```python
from build123d import *

# Parameters (mm, degrees)
BOSS_EXTRUDE1_DEPTH = 1.524


with BuildPart() as part:
    # Sketch1 → Boss-Extrude1 (new body)
    with BuildSketch(Plane.XY):
        with BuildLine():
            ThreePointArc((12.566304874, -9.8933052), (12.77131161, -10.004957793), (12.965201909, -10.13496016))
            ThreePointArc((12.965201909, -10.13496016), (18.14143902, -15.472865183), (21.320013307, -22.194719552))
            ThreePointArc((21.320013307, -22.194719552), (20.806583347, -23.173609324), (19.854339012, -22.612301713))
            ThreePointArc((19.854339012, -22.612301713), (16.93227249, -16.403886417), (12.182265789, -11.452085777))
            ThreePointArc((12.182265789, -11.452085777), (11.989118214, -11.3205608), (11.784700698, -11.207342939))
            ThreePointArc((11.784700698, -11.207342939), (5.914450191, -6.588756496), (2.396003148, 0))
            Line((2.396003148, 0), (3.20554689, 0))
            Line((3.20554689, 0), (3.20554689, 1.524))
            Line((3.20554689, 1.524), (4.72954689, 1.524))
            Line((4.72954689, 1.524), (4.72954689, 0))
            Line((4.72954689, 0), (5.480406076, 0))
            ThreePointArc((5.480406076, 0), (5.996385034, -3.275905029), (7.587657532, -6.185482298))
            ThreePointArc((7.587657532, -6.185482298), (9.902770623, -8.273313508), (12.566304874, -9.8933052))
        make_face()
    extrude(amount=BOSS_EXTRUDE1_DEPTH)


solid = part.part
```
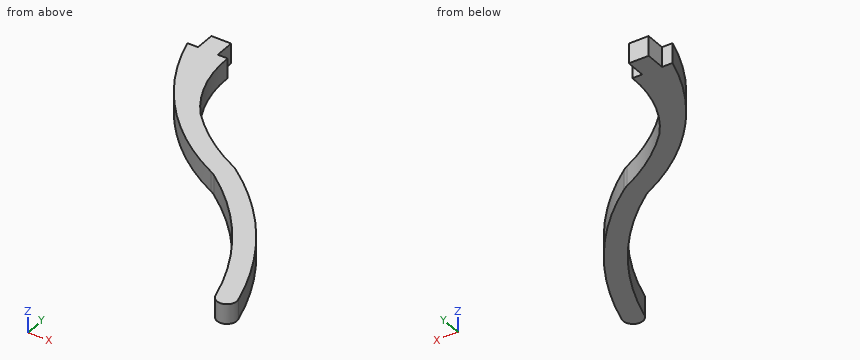
CAD build for the part. Positions are in the model's coordinates, mm. Coordinates: 2 decimals unless noted, no trailing zeros. Order: outer loops, then holes, each group sorted by start corner. A loop starts at its lowest first (then second) coordinate and runs counter-clockwise, first axis right, second up.
(1) Saw through at C-C, the plane y = -18.5. Write the cut outline in (x, z), and give its area (3 significant figures).
Solution:
outline: (18.2, 0) - (19.91, 0) - (19.91, 1.52) - (18.2, 1.52) - close
area: 2.60 mm2
(2) Saw through at A-A, the plane z = 0.5. Write the cut outline in (x, y), and give its area (3 significant figures).
Solution:
outline: (2.4, 0) arc R18.18 ccw to (11.78, -11.21) arc R2.54 cw to (12.18, -11.45) arc R21.23 cw to (19.85, -22.61) arc R0.76 ccw (long way) to (21.32, -22.19) arc R22.75 ccw to (12.97, -10.13) arc R2.54 ccw to (12.57, -9.89) arc R16.66 cw to (7.59, -6.19) arc R9.68 cw to (5.48, 0) - (4.73, 0) - (4.73, 1.52) - (3.21, 1.52) - (3.21, 0) - close
area: 51.6 mm2
(3) Pin check, flat tips, straight feed: pin 1 Ø0.9 at (x, z) = (2.5, 0.5) entering from +Y; pin 2 Ø0.8 at (y, z) = (1, 0.5) entering from +X. Stop position of each tip, or through.
Solution:
pin 1: stops at y = 0
pin 2: stops at x = 4.73
(4) Drill centre lines: L1, parallel to X at y = -18.5, z = 1.4; L2, parallel to Y at x = 13.5, z = 0.6; L3, parallel to X at y = -10.25, z = 1.4. Where is each one in solid material? Low to high.
Solution:
L1: x = 18.2 to 19.91
L2: y = -12.53 to -10.54
L3: x = 10.09 to 13.12
(5) Saw through at B-B, the plane x = 13.75. Write the cut outline in (y, z), and give its area (3 significant figures).
Solution:
outline: (-12.75, 0) - (-10.74, 0) - (-10.74, 1.52) - (-12.75, 1.52) - close
area: 3.06 mm2
